The listing builds one solid part. Answer for the finished solid, in the listing's coordinates (mm). A direction names the side the tool comes from. Round coordinates to 2 decimals unless told otherwise and drop trailing zeros. Loops run counter-clockwise (first coordinate to the right, second up) from the corner with the lowest first, then second, coordinate; pieces in that order, holes last. Notation, with made-up numbers: (82, -4) -> (137, -4) arc R14 ccw to (137, 0) -> close; hole circle Ø2 at (69.25, 63). An arc over 180 degrees is marked (long way). Answer in a Markdown table with one row per item. Add a question column.
```python
from build123d import *

# Parameters (mm, degrees)
CHANFREIN2_SIZE              = 0.5
R_P_TITION_CIRCULAIRE1_COUNT = 3


with BuildPart() as part:
    # Esquisse1 → Base-Révolution (revolve)
    with BuildSketch(Plane.XY, mode=Mode.PRIVATE) as base_r_volution_sk:
        with BuildLine():
            Line((-33, 0), (-33, 6))
            Line((-33, 6), (-11, 6))
            Line((-11, 6), (-11, 8))
            Line((-11, 8), (-10, 8))
            ThreePointArc((-10, 8), (-7.878679656, 8.878679656), (-7, 11))
            Line((-7, 11), (-7, 24))
            Line((-7, 24), (0, 24))
            Line((0, 24), (0, 6))
            Line((0, 6), (-4, 6))
            Line((-4, 6), (-4, 3.464101615))
            Line((-4, 3.464101615), (-6, 0))
            Line((-6, 0), (-33, 0))
        make_face()
    revolve(base_r_volution_sk.sketch.rotate(Axis((0, 0, 0), (-1, 0, 0)), 90), axis=Axis((0, 0, 0), (-1, 0, 0)))

    # Chanfrein2
    chanfrein2_edges = [part.edges().sort_by_distance(p)[0] for p in [
        (0, 0, 24),
        (-7, 0, 24),
    ]]
    chamfer(chanfrein2_edges, length=CHANFREIN2_SIZE)

    # Esquisse2 → Boss.-Révol.1 (revolve)
    with BuildSketch(Plane.XY):
        Polygon((-28, 3), (-33, 3), (-34, 2), (-51, 2), (-52, 1), (-52, -1.5), (-28, -1.5), align=None)
    revolve(axis=Axis((-19, -1.5, 0), (-1, 0, 0)))

    # Esquisse3 → Enlèvement de matière-Révolution2 (revolve, cut)
    with BuildSketch(Plane.XY, mode=Mode.PRIVATE) as enl_vement_de_mati_re_r_volution2_sk:
        Polygon((-8, 23), (-3, 23), (-3, 21), (4, 21), (4, 18), (-8, 18), align=None)
    enl_vement_de_mati_re_r_volution2 = revolve(enl_vement_de_mati_re_r_volution2_sk.sketch.rotate(Axis((-12, 18, 0), (1, 0, 0)), 90), axis=Axis((-12, 18, 0), (1, 0, 0)), mode=Mode.SUBTRACT)

    # Répétition circulaire1: Enlèvement de matière-Révolution2 ×3 about axis
    r_p_tition_circulaire1_axis = Axis((0, 0, 0), (1, 0, 0))
    for i in range(1, R_P_TITION_CIRCULAIRE1_COUNT):
        add(enl_vement_de_mati_re_r_volution2.rotate(r_p_tition_circulaire1_axis, i * 360 / R_P_TITION_CIRCULAIRE1_COUNT), mode=Mode.SUBTRACT)


solid = part.part
```
Item 1: Section A-A, the plane x = -47 is taken. Write down the section's boundary in (y, z), and give its area (3 significant figures).
Item 2: The mould has two halves that part along Z. Classify faces 1 (the cylindrical face through (-1.48, -9.13, 12.59)), 2 (the cylindrical face through (-21.846, -1.802, -5.723)), 3 (the flat face through (-11, -6, -2)), 4 (the flat face through (-3, -12, 14)): +Z half, -Z half, draft (parallel to the pull), parting line (faces both ways), or undercut.
Item 3: Consider L1, parallel to Y at x = -1.3, z = 0; L2, parallel to Y at x = -4.9, z = 0; L3, parallel to Z at x = -3.5, y = -10.5. Determine where each line is inside the solid, lowest interval first. Write a range as from..to.
Item 4: Flat-ended cylindrical pins translate along their axes: P1, Ø3, axis at y = 18.5, z = -1.5, coming from the -X side; P2, Ø10, axis at x = -21.5, y = 2, coming from the -Z side; P3, Ø1, axis at x = -6.5, z = 17.5, coming from the +Y side. Find the tip coordinate at first contact, or state that the pin passes through.
Item 5: Section B-B, the plane x = -29.5 is taken. Write down the section's boundary in (y, z), and give its area (3 significant figures).
Item 6: For faces 5 (the cylindrical face through (-10.49, 7.81, 1.73)), 6 (the cylindrical face through (-2.028, -1.802, -5.723)), 7 (the cylindrical face through (-1.48, -6.34, -14.2)), determine the directions among +Z, -Z, +X, -X, +Y, -Y from which every point of the face is accessible in a straight line to the end or side of a thin tool.
Here are the results:
| question | item | result |
|---|---|---|
| 1 | outline | circle Ø7 at (-1.5, 0) |
| 1 | area | 38.5 mm² |
| 2 | face 1 | undercut |
| 2 | face 2 | parting line |
| 2 | face 3 | draft |
| 2 | face 4 | undercut |
| 3 | L1 | y = -24..-6, 6..15, 21..24 |
| 3 | L2 | y = -24..-1.91, 1.91..13, 23..24 |
| 3 | L3 | z = -21.58..-20.36, -10.82..10.82, 20.36..21.58 |
| 4 | P1 | stops at x = -3 |
| 4 | P2 | stops at z = -6 |
| 4 | P3 | stops at y = 16.94 |
| 5 | outline | circle Ø12 at (0, 0) |
| 5 | area | 113 mm² |
| 6 | face 5 | -X |
| 6 | face 6 | +X |
| 6 | face 7 | +X, -X |
